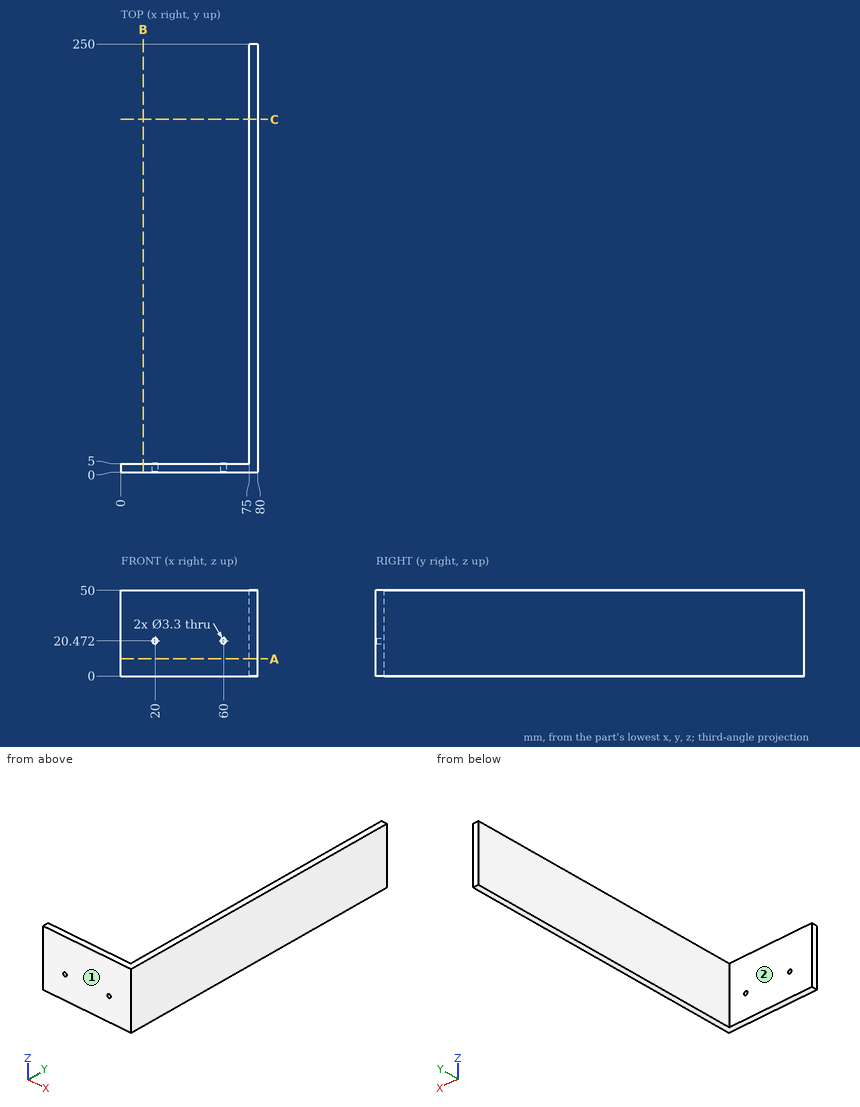
Source: three-view drawing plus pictorial views. Frame: mm from the lowest corner of the part. A direction names the side the tool comes from. Coordinates: 2 decimals unless noted, no trailing zeros. Write each loop counter-clockwise with the first axis right and the second up, starting at its lowest first coordinate (ties: lowest second). Pieces come first, ordered by that corner, then holes. Notation, with made-up numbers: (-1.75, 83.5) - (30.25, 83.5) arc R19 cw to (30.25, 89.5) - close; hole circle Ø7 at (17.25, 65). An arc over 180 degrees is marked (long way). Return JSON: item names as keys, results as strings.
Item 1: Section query C-C (y = 206). Output: boundary loops of the cut face in (x, z), and give its area (3 significant figures).
Completed:
{"outline": "(75, 0) - (80, 0) - (80, 50) - (75, 50) - close", "area": "250 mm2"}
Item 2: Pin query (flat end, axial travel): pin 1 Ø5 at (x, z) = (52.5, 39) entering from +Y; pin 2 Ø4 at (y, z) = (119.5, 38.5) entering from -X. Return the tip coordinate at first contact, or that it passes through.
Completed:
{"pin 1": "stops at y = 5", "pin 2": "stops at x = 75"}
Item 3: Section query A-A (z = 10). Output: boundary loops of the cut face in (x, y), and give its area (4 significant figures).
Completed:
{"outline": "(0, 0) - (80, 0) - (80, 250) - (75, 250) - (75, 5) - (0, 5) - close", "area": "1,625 mm2"}
Item 4: Line query: L1, parallel to Z at x = 60, y = 3.55; L2, parallel to Y at x = 28.5, z = 20.5; L3, parallel to X at y = 103.5, z = 19. Output: solid intervals per line, ascending.
Completed:
{"L1": "z = 0 to 18.82, 22.12 to 50", "L2": "y = 0 to 5", "L3": "x = 75 to 80"}
Item 5: Reachability of the marked faces 1 and 2 from +Z, -Z, +X, -X, +Y, -Y: full face, straight path, thin tool, end or side. Return the list, or none.
Completed:
{"face 1": "+Z, -Z, +X, -X, -Y", "face 2": "+Z, -Z, -X, +Y"}
Item 6: Section query B-B (x = 13). Output: boundary loops of the cut face in (y, z).
Completed:
{"outline": "(0, 0) - (5, 0) - (5, 50) - (0, 50) - close"}
